Job drawing, mm, ordinate dimensions from the low corner. One solid piece. Give positions to 0.01 mm unless a question says otherwise; leave off trailing zeros. Order: outer loops, then holes, each group sorted by start corner. A loop starts at its lowest first (then second) coordinate and runs counter-clockwise, first axis right, second up. Notation, with made-up numbers: M 30,34 L 43,34 A17 cw 43,48 Z; hole C 43.5,47.5 d9. An arc over 180 degrees is marked long. One line per item, written item: value. Start each with the question number.
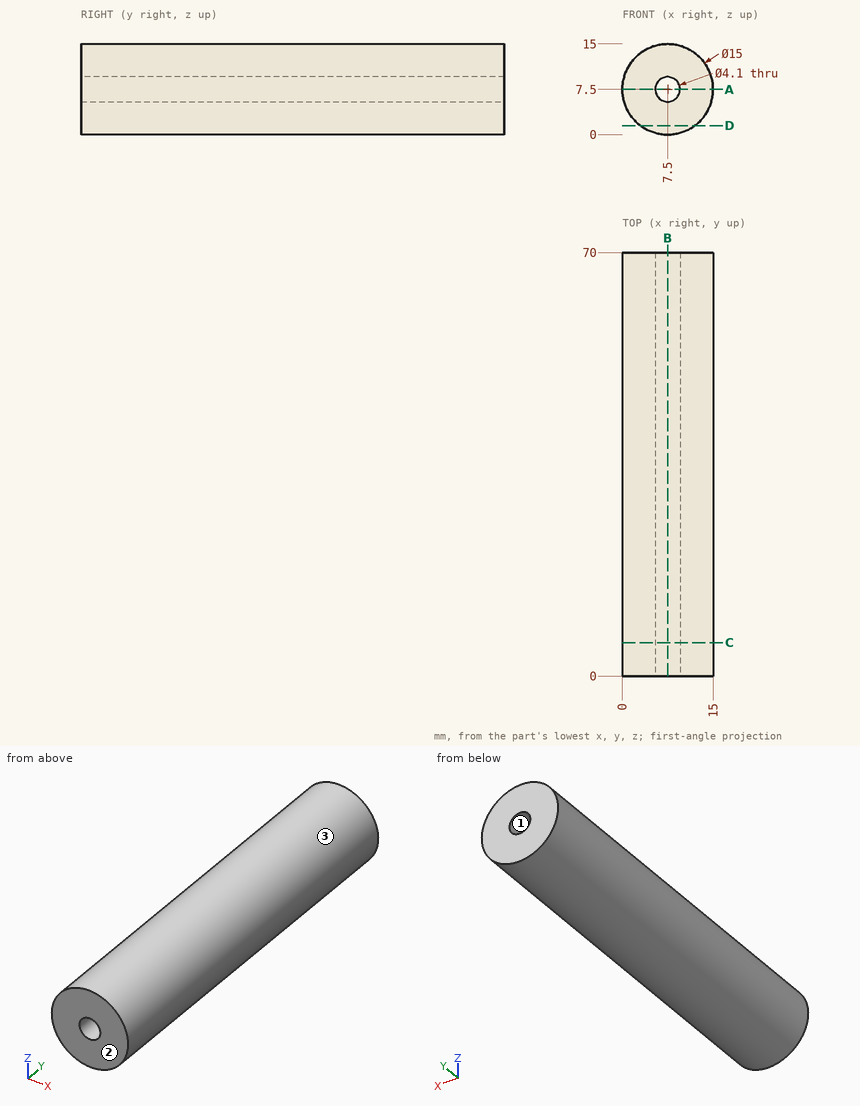
1) Drill centre lines: line 1 (X direction, y = 32, z = 7.5); line 2 (X direction, y = 56, z = 9); line 3 (X direction, y = 48.5, z = 11). Where is each one in solid material? Low to high.
2) Pull direction Z, two halves, no side cores. Call the marked faces 1, 2 and 3: pulls with the +Z half, pulls with the -Z half, needs draft (parallel to the pull), parting line crosses it, or undercut.
3) Slice it at D-D (z = 1.5). List the corners of the cut face in (x, y), plus the area to 3 significant figures.
4) Slice it at C-C (y = 5.5). List the corners of the cut face in (x, z), plus the area to 3 significant figures.
5) Drop flat-ended pins along their axis: P1, Ø4, axis at y = 49.5, z = 5, coming from the -X side; P2, Ø1, axis at y = 24, z = 5.5, coming from the +X side; P3, Ø1, axis at x = 8, z = 12, coming from the -Y side; P4, Ø1, axis at x = 4, y = 14.5, coming from the -Z side. Give the stop position or say it passes through.
6) Slice it at A-A (z = 7.5). List the corners of the cut face in (x, y).
7) Slice it at B-B (x = 7.5). List the corners of the cut face in (y, z), plus the area to 3 significant figures.
Results list:
1. line 1: x = 0 to 5.45, 9.55 to 15
1. line 2: x = 0.15 to 6.1, 8.9 to 14.85
1. line 3: x = 0.87 to 14.13
2. face 1: undercut
2. face 2: needs draft
2. face 3: parting line crosses it
3. outline: M 3,0 L 12,0 L 12,70 L 3,70 Z
3. area: 630 mm²
4. outline: C 7.5,7.5 d15; hole C 7.5,7.5 d4.1
4. area: 164 mm²
5. P1: stops at x = 0.02
5. P2: stops at x = 14.85
5. P3: stops at y = 0
5. P4: stops at z = 0.63
6. outline: M 0,0 L 5.45,0 L 5.45,70 L 0,70 Z; M 9.55,0 L 15,0 L 15,70 L 9.55,70 Z
7. outline: M 0,0 L 70,0 L 70,5.45 L 0,5.45 Z; M 0,9.55 L 70,9.55 L 70,15 L 0,15 Z
7. area: 763 mm²
